Here's how the part is built. I have some questions about the finished solid (model axes, mm). A direction names the side the tool comes from. Round coordinates to 2 decimals unless told otherwise and drop trailing zeros. Loops run counter-clockwise (first coordinate to the right, second up) from the corner with the lowest first, then second, coordinate; pieces in that order, holes last. Notation, with made-up numbers: (30.25, -6) - (62.25, -6) arc R16 ccw to (62.25, 3) - close; hole circle Ø1 at (49.5, 2.25). An arc over 180 degrees is marked (long way). Answer as a JSON object with one key per item and string values. Group by question number.
1) If I drill on line 1 along X through (y, z) = (-1.9, 2.5); line 2 along Z through (x, y) = (0, -0.9); line 3 along Z through (x, y) = (-15, -0.6), over which ranges is the centre line in solid material (lowest first)? Write a range as [from, to].
2) If we mould it in two halves opening along X, with no side actions, what happens to faces 5 (the face through (8, -1, 20)), 6 (the face through (3.85, -1, -20)), 7 (the face through (10.994, -1.232, 19.624))? For each: pulls with the +X half, pulls with the -X half, needs draft (parallel to the pull), parting line crosses it, or undercut.
3) I want a section at A-A, the plane z = -19.5. Please give me the cut outline in (x, y).
4) Will these pins go through, and if not, where does the flat tip stop? P1, Ø0.8, axis at x = -14.5, y = -1, coming from the -Z side; P2, Ø1.2, axis at x = 13.5, y = -0.5, coming from the +Z side; P3, Ø0.8, axis at y = -1.5, z = -20.5, coming from the -X side.
5) I want a section at B-B, the plane x = 0. Please give me the cut outline in (y, z).
6) Which directions (+Z, -Z, +X, -X, +Y, -Y) give clear straight access to the entire face, cutting with the end or side of a thin tool? Please do faces 1 (the face through (0, -1, -17.5)), 2 (the face through (-4.206, -1.232, 19.624)), 3 (the face through (-11.35, -1, 18)), 4 (the face through (-11.35, -1, -20)).
from build123d import *

# Parameters (mm, degrees)
F1_DEPTH = 2.5


with BuildPart() as f1:
    # F0 (on Front) → F1 (new body)
    with BuildSketch(Plane.XZ):
        with BuildLine():
            Line((-11.35, 17.5), (-16.8, 17.5))
            Line((-16.8, 17.5), (-16.8, 2.5))
            Line((-16.8, 2.5), (-9, 2.5))
            ThreePointArc((-9, 2.5), (0, 11.5), (9, 2.5))
            Line((9, 2.5), (16.8, 2.5))
            Line((16.8, 2.5), (16.8, 17.5))
            Line((16.8, 17.5), (11.35, 17.5))
            Line((11.35, 17.5), (11.35, 18.75))
            ThreePointArc((11.35, 18.75), (10.983883, 19.633883), (10.1, 20))
            Line((10.1, 20), (5.1, 20))
            ThreePointArc((5.1, 20), (4.216117, 19.633883), (3.85, 18.75))
            Line((3.85, 18.75), (3.85, 17.5))
            Line((3.85, 17.5), (-3.85, 17.5))
            Line((-3.85, 17.5), (-3.85, 18.75))
            ThreePointArc((-3.85, 18.75), (-4.216117, 19.633883), (-5.1, 20))
            Line((-5.1, 20), (-10.1, 20))
            ThreePointArc((-10.1, 20), (-10.983883, 19.633883), (-11.35, 18.75))
            Line((-11.35, 18.75), (-11.35, 17.5))
        make_face()
        with BuildLine():
            Line((-9, 2.5), (-16.8, 2.5))
            Line((-16.8, 2.5), (-16.8, -17.5))
            Line((-16.8, -17.5), (-11.35, -17.5))
            Line((-11.35, -17.5), (-11.35, -22.25))
            ThreePointArc((-11.35, -22.25), (-10.983883, -23.133883), (-10.1, -23.5))
            Line((-10.1, -23.5), (-5.1, -23.5))
            ThreePointArc((-5.1, -23.5), (-4.216117, -23.133883), (-3.85, -22.25))
            Line((-3.85, -22.25), (-3.85, -17.5))
            Line((-3.85, -17.5), (3.85, -17.5))
            Line((3.85, -17.5), (3.85, -22.25))
            ThreePointArc((3.85, -22.25), (4.216117, -23.133883), (5.1, -23.5))
            Line((5.1, -23.5), (10.1, -23.5))
            ThreePointArc((10.1, -23.5), (10.983883, -23.133883), (11.35, -22.25))
            Line((11.35, -22.25), (11.35, -17.5))
            Line((11.35, -17.5), (16.8, -17.5))
            Line((16.8, -17.5), (16.8, 2.5))
            Line((16.8, 2.5), (9, 2.5))
            ThreePointArc((9, 2.5), (0, -6.5), (-9, 2.5))
        make_face()
    extrude(amount=F1_DEPTH)


solid = f1.part
Outcome:
{
 "1": {"line 1": "[-16.8, -9], [9, 16.8]", "line 2": "[-17.5, -6.5], [11.5, 17.5]", "line 3": "[-17.5, 17.5]"},
 "2": {"face 5": "needs draft", "face 6": "undercut", "face 7": "pulls with the +X half"},
 "3": {"outline": "(-11.35, -2.5) - (-3.85, -2.5) - (-3.85, 0) - (-11.35, 0) - close; (3.85, -2.5) - (11.35, -2.5) - (11.35, 0) - (3.85, 0) - close"},
 "4": {"P1": "z = -17.5", "P2": "z = 17.5", "P3": "x = -11.35"},
 "5": {"outline": "(-2.5, -17.5) - (0, -17.5) - (0, -6.5) - (-2.5, -6.5) - close; (-2.5, 11.5) - (0, 11.5) - (0, 17.5) - (-2.5, 17.5) - close"},
 "6": {"face 1": "-Z, +Y, -Y", "face 2": "+Z, +Y, -Y", "face 3": "+Z, -X, +Y, -Y", "face 4": "-Z, -X, +Y, -Y"}
}
